Autodesk Inventor part; units mm, degrees
ref_plane "YZ Plane" through (0, 0, 0) normal (1, 0, 0) x (0, 1, 0)
ref_plane "XZ Plane" through (0, 0, 0) normal (0, 1, 0) x (-1, 0, 0)
ref_plane "XY Plane" through (0, 0, 0) normal (0, 0, 1) x (1, 0, 0)
sketch "スケッチ1" plane through (0, 0, 0) normal (0, 0, 1) x (1, 0, 0)
  line L0 (-10, 17) -> (0, 17)
  line L1 (0, 17) -> (0, 15)
  line L2 (0, 15) -> (-10, 15)
  line L3 (-10, 15) -> (-10, 17)
  line L4 (0, -3.4) -> (0, 20.4)
  point P0 (0, 0)
  dimension "d0" = 10
  dimension "d1" = 2
  dimension "d2" = 15
extrude "押し出し1" add sketch "スケッチ1" along normal blind 5
sketch "スケッチ2" plane through (0, 0, 5) normal (0, 0, 1) x (1, 0, 0)
  line L0 (0, 17) -> (-10, 17)
  line L1 (-10, 17) -> (-8.5, 17)
  line L2 (-8.5, 17) -> (-8.5, 0)
  line L3 (-8.5, 0) -> (-10, 0)
  line L4 (-10, 0) -> (-10, 17)
  line L5 (-10, 15) -> (0, 15)
  line L6 (0, 15) -> (0, 17)
  line L7 (0, 17) -> (-10, 17)
  line L8 (-10, 17) -> (-10, 15)
  point P0 (0, 0)
  point P1 (-8.5, 15)
  dimension "d5" = 1.5
extrude "押し出し2" add sketch "スケッチ2" along normal blind 10
sketch "スケッチ3" plane through (-8.5, 0, 5) normal (1, 0, 0) x (0, 0, -1)
  line L0 (-7.5, 12) -> (-2.5, 12)
  line L1 (-2.5, 12) -> (-2.5, 2)
  line L2 (-2.5, 2) -> (-7.5, 2)
  line L3 (-7.5, 2) -> (-7.5, 12)
  line L4 (0, 0) -> (-10, 0)
  line L5 (0, 15) -> (-10, 15)
  point P0 (5, 0)
  point P1 (-5, 2)
  point P2 (-5, 0)
  dimension "d8" = 2
  dimension "d9" = 5
  dimension "d13" = 3
extrude "押し出し3" cut sketch "スケッチ3" against normal through all
fillet "フィレット1" radius 3 1 edges at (-8.5, 15, 10)
mirror "ミラー1" about plane through (0, 15, 0) normal (1, 0, 0)
mirror "ミラー2" about plane through (-5, 16, 0) normal (0, 0, -1)
sketch "スケッチ4" plane through (0, 0, 15) normal (0, 0, 1) x (1, 0, 0)
  line L0 (-10, 17) -> (-10, 0)
  line L1 (-10, 17) -> (-34, 17)
  line L2 (-34, 17) -> (-34, 13)
  line L3 (-34, 13) -> (-10, 13)
  line L4 (-10, 13) -> (-10, 17)
  line L5 (-34, 17) -> (-31, 17)
  line L6 (-31, 17) -> (-31, 2)
  line L7 (-31, 2) -> (-34, 2)
  line L8 (-34, 2) -> (-34, 17)
  point P0 (0, 0)
  point P1 (-31, 13)
  dimension "d14" = 4
  dimension "d15" = 3
  dimension "d16" = 21
  dimension "d17" = 15
extrude "押し出し4" add sketch "スケッチ4" against normal up to surface (30 mm away)
fillet "フィレット2" radius 2 1 edges at (-34, 17, 0)
properties part number "connetcor_female_cover"
Source: CAD feature listing. Evaluate the final solid. Frame: model axes, mm. A direction names the side the tool comes from. Give positions to 0.01 mm unless a question says otherwise; leave off trailing zeros. Write each loop counter-clockwise with the first axis right and the second up, starting at its lowest first coordinate (ties: lowest second). Pieces come first, ordered by that corner, then holes. Notation, with made-up numbers: (80.25, 87.25) - (108.25, 87.25) arc R31 ccw to (108.25, 113.25) - close; hole circle Ø9 at (28, 35.25). An arc over 180 degrees is marked (long way). One line per item, written item: value. Start each with the question number.
Q1. Section query C-C, the plane z = -3.75. Return the cut outline in (x, y), then the cut area to 3 significant figures.
Q2. Section query A-A, the plane z = 10.5. Count the separate pieces of the cut face and the enclosed holes in it, then the cut area to 3 significant figures.
Q3. Set-up query: faces 1 (the face through (-32, 2, 0)), 2 (the face through (9, 2, -10)), 3 (the face through (9, 8, 5)), 4 (the face through (0, 15, 0)), 5 (the face through (-10, 6, 7)). Return all of +Z, -Z, +X, -X, +Y, -Y with unobstructed straight access to the full face (end or side cutting, diameter ignored); none if empty.
Q4. First-contact query: pin 1 Ø1.5 at (y, z) = (9.5, 1) entering from +X; pin 2 Ø1.5 at (x, z) = (-22.5, -3.5) entering from -Y; pin 3 Ø2 at (x, y) = (-7, 7.5) entering from -Z; pin 4 Ø10 at (x, z) = (-1, 7) entering from -Y. Flat tips, straight axial feed; report the tip coordinate or a pass-through.
Q5. Section query D-D, the plane y = 13.75. Return the cut outline in (x, z), then the cut area to 3 significant figures.
Q6. Material intervals for probe 1 along X at (y, z) = (7.5, 5.75); probe 2 along X at (y, z) = (1, 12); probe 3 along X at (y, z) = (14, -2.5), sorted ascending. Write a range as from..to.
Q7. Draft query along Y for faces 6 (the face through (-9, 12, 10)), 7 (the face through (9, 7, 7.5)), 8 (the face through (10, 16, 0)), 9 (the face through (7.6, 14.14, -10.07)). Return one class per face: +Y half, -Y half, draft (parallel to the pull), parting line (faces both ways), or undercut.
Answer:
1. outline: (-34, 2) - (-31, 2) - (-31, 13) - (-10, 13) - (-10, 15) - (10, 15) - (10, 17) - (-32, 17) arc R2 ccw to (-34, 15) - close
1. area: 168 mm2
2. separate pieces: 3
2. enclosed holes: 0
2. area: 187 mm2
3. face 1: +Z, -Z, -X, -Y
3. face 2: +X
3. face 3: +X, -Y
3. face 4: -Y
3. face 5: +Z, -Z, -Y
4. pin 1: stops at x = -31
4. pin 2: stops at y = 13
4. pin 3: passes through
4. pin 4: stops at y = 14.96
5. outline: (-34, -15) - (-7.94, -15) - (-7.94, -5) - (-10, -5) - (-10, 5) - (-7.94, 5) - (-7.94, 15) - (-34, 15) - close; (7.94, -15) - (10, -15) - (10, -5) - (7.94, -5) - close; (7.94, 5) - (10, 5) - (10, 15) - (7.94, 15) - close
5. area: 803 mm2
6. probe 1: x = -34..-31, -10..-8.5, 8.5..10
6. probe 2: x = -10..-8.5, 8.5..10
6. probe 3: x = -34..-10
7. face 6: undercut
7. face 7: undercut
7. face 8: draft
7. face 9: -Y half
